```python
from build123d import *

# Parameters (mm, degrees)
SKETCH1_W            = 19.05
SKETCH1_H            = 19.05
BOSS_EXTRUDE1_DEPTH  = 5.08
M3_CLEARANCE_HOLE1_D = 3.4
CUT_EXTRUDE2_DEPTH   = 3.175


with BuildPart() as part:
    # Sketch1 → Boss-Extrude1 (new body)
    with BuildSketch(Plane(origin=(0, 0, 0), x_dir=(1, 0, 0), z_dir=(0, 1, 0))):
        Rectangle(SKETCH1_W, SKETCH1_H)
    extrude(amount=BOSS_EXTRUDE1_DEPTH)

    # M3 Clearance Hole1 (through all)
    with Locations(Plane(origin=(0, 0, 0), x_dir=(-1, 0, 0), z_dir=(0, -1, 0))):
        with Locations((-4.445, 0), (4.445, 0)):
            Hole(M3_CLEARANCE_HOLE1_D / 2)

    # Sketch8 → Cut-Extrude2 (cut)
    with BuildSketch(Plane.XZ):
        Polygon((-7.239, -1.613116652), (-4.445, -3.226233304), (-1.651, -1.613116652), (-1.651, 1.613116652), (-4.445, 3.226233304), (-7.239, 1.613116652), align=None)
        Polygon((7.239, -1.613116652), (7.239, 1.613116652), (4.445, 3.226233304), (1.651, 1.613116652), (1.651, -1.613116652), (4.445, -3.226233304), align=None)
    extrude(amount=-CUT_EXTRUDE2_DEPTH, mode=Mode.SUBTRACT)


solid = part.part
```
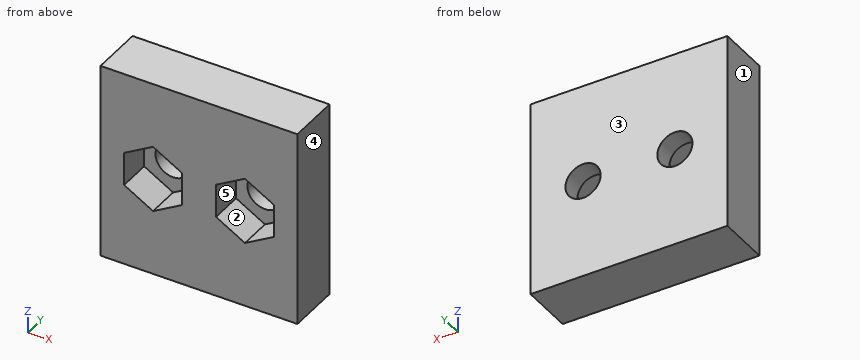
Verification items for the finished model (mm, model axes). Face numbers are marked on the shaded views. A direction names the side the tool comes from. Coordinates: 2 decimals unless noted, no trailing zeros. Loops run counter-clockwise (first coordinate to the right, second up) from the corner with the lowest first, then second, coordinate; pieces in that order, holes last. Notation, with made-up numbers: (48, 46) - (77, 46) arc R25 cw to (77, 65) - close; hole circle Ø9 at (57, -16). An arc over 180 degrees is marked (long way). Return JSON: item names as keys, results as strings.
1. Tool access check on the marked faces 4 and 5. Record the directions out of +Z, -Z, +X, -X, +Y, -Y that give a thin tool (end or side, any length) a straight path to the whole face; none if there is none.
Established:
{"face 4": "+Z, -Z, +X, +Y, -Y", "face 5": "-Y"}
2. Thickness scan on L1, parallel to X at y = 1.05, z = 1.5 (3 decimals); L2, parallel to Z at x = 5, y = 3.7 (3 decimals); L3, parallel to X at y = 2.25, z = -2.5 (3 decimals). Record the ranges inside material, lowest first.
Established:
{"L1": "x = -9.525 to -7.239, -1.651 to 1.651, 7.239 to 9.525", "L2": "z = -9.525 to -1.607, 1.607 to 9.525", "L3": "x = -9.525 to -5.703, -3.187 to 3.187, 5.703 to 9.525"}
3. Section check D-D, the plane z = 2.25. Record the boundary of the cut face in (x, y) (3 decimals), then the cut area to 3 significant figures.
Established:
{"outline": "(-9.525, 0) - (-6.136, 0) - (-6.136, 3.175) - (-2.754, 3.175) - (-2.754, 0) - (2.754, 0) - (2.754, 3.175) - (6.136, 3.175) - (6.136, 0) - (9.525, 0) - (9.525, 5.08) - (-9.525, 5.08) - close", "area": "75.3 mm2"}
4. Mould release check, pull along X, two halves, no side actions. Record for the marked faces 1, 2 and 3: +X half, -X half, draft (parallel to the pull), parting line (faces both ways), or undercut.
Established:
{"face 1": "-X half", "face 2": "undercut", "face 3": "draft"}
5. Section check C-C, the plane y = 2.2. Record the boundary of the cut face in (x, z) (3 decimals).
Established:
{"outline": "(-9.525, -9.525) - (9.525, -9.525) - (9.525, 9.525) - (-9.525, 9.525) - close; hole (-7.239, -1.613) - (-4.445, -3.226) - (-1.651, -1.613) - (-1.651, 1.613) - (-4.445, 3.226) - (-7.239, 1.613) - close; hole (1.651, -1.613) - (4.445, -3.226) - (7.239, -1.613) - (7.239, 1.613) - (4.445, 3.226) - (1.651, 1.613) - close"}
6. Section check B-B, the plane x = -3.25. Record the boundary of the cut face in (y, z) (3 decimals), then the cut area to 3 significant figures.
Established:
{"outline": "(0, -9.525) - (5.08, -9.525) - (5.08, -1.209) - (3.175, -1.209) - (3.175, -2.536) - (0, -2.536) - close; (0, 2.536) - (3.175, 2.536) - (3.175, 1.209) - (5.08, 1.209) - (5.08, 9.525) - (0, 9.525) - close", "area": "76.1 mm2"}
7. Section check A-A, the plane z = 0. Record the boundary of the cut face in (x, y) (3 decimals).
Established:
{"outline": "(-9.525, 0) - (-7.239, 0) - (-7.239, 3.175) - (-6.145, 3.175) - (-6.145, 5.08) - (-9.525, 5.08) - close; (-2.745, 3.175) - (-1.651, 3.175) - (-1.651, 0) - (1.651, 0) - (1.651, 3.175) - (2.745, 3.175) - (2.745, 5.08) - (-2.745, 5.08) - close; (6.145, 3.175) - (7.239, 3.175) - (7.239, 0) - (9.525, 0) - (9.525, 5.08) - (6.145, 5.08) - close"}
